Autodesk Inventor part; units mm, degrees
ref_plane "YZ Plane" through (0, 0, 0) normal (1, 0, 0) x (0, 1, 0)
ref_plane "XZ Plane" through (0, 0, 0) normal (0, 1, 0) x (-1, 0, 0)
ref_plane "XY Plane" through (0, 0, 0) normal (0, 0, 1) x (1, 0, 0)
sketch "Эскиз1" plane through (0, 0, 0) normal (1, 0, 0) x (0, 1, 0)
  circle A0 centre (8.3565, 10.4457) radius 25
  point P0 (0, 0)
  dimension "d0" = 50
extrude "Выдавливание1" add sketch "Эскиз1" along normal blind 15
sketch "Эскиз2" plane through (0, 8.3565, 10.4457) normal (-1, 0, 0) x (0, 0, 1)
  circle A0 centre (0, 0) radius 22.5
  point P0 (-10.4457, -8.3565)
  dimension "d3" = 45
extrude "Выдавливание2" cut sketch "Эскиз2" against normal blind 5
sketch "Эскиз3" plane through (15, 8.3565, 10.4457) normal (1, 0, 0) x (0, 0, -1)
  circle A0 centre (0, 0) radius 22.5
  point P0 (10.4457, -8.3565)
  dimension "d6" = 45
extrude "Выдавливание3" cut sketch "Эскиз3" against normal blind 5
sketch "Эскиз7" plane through (5, 8.3565, 10.4457) normal (-1, 0, 0) x (0, 0, 1)
  circle A0 centre (0, 0) radius 5
  line L0 (5, 0) -> (-5, 0)
  line L1 (-5, 0) -> (-5, 30.8448)
  line L2 (-5, 30.8448) -> (5, 30.8448)
  line L3 (5, 30.8448) -> (5, 0)
  line L4 (5, 0) -> (-5, 0)
  line L5 (-5, 0) -> (-5, -27.2335)
  line L6 (-5, -27.2335) -> (5, -27.2335)
  line L7 (5, -27.2335) -> (5, 0)
  line L8 (0, -5) -> (31.8043, -5)
  line L9 (31.8043, -5) -> (31.8043, 5)
  line L10 (31.8043, 5) -> (0, 5)
  line L11 (0, 5) -> (0, -5)
  line L12 (0, -5) -> (-27.8953, -5)
  line L13 (-27.8953, -5) -> (-27.8953, 5)
  line L14 (-27.8953, 5) -> (0, 5)
  line L15 (0, 5) -> (0, -5)
  circle A1 centre (0, 0) radius 22.5
  circle A2 centre (0, 0) radius 17.5
  point P0 (-10.4457, -8.3565)
  point P1 (5, -16.7705)
  point P2 (16.7705, -5)
  point P3 (5, -5)
  point P4 (-16.7705, -5)
  point P5 (-5, -16.7705)
  point P6 (-5, -5)
  point P7 (16.7705, 5)
  point P8 (5, 16.7705)
  point P9 (5, 5)
  point P10 (-5, 16.7705)
  point P11 (-16.7705, 5)
  point P12 (-5, 5)
  dimension "d13" = 10
  dimension "d14" = 35
extrude "Выдавливание4" cut sketch "Эскиз7" against normal blind 10 contours L3 A2 L10 | L8 A2 L7 | L14 A2 L1 | L5 A2 L12
fillet "Сопряжение1" radius 1 2 edges at (15, -16.6435, 10.4457) (0, -16.6435, 10.4457)
properties part number "колесо" material "Пластик САН"
For this review, take the finished solid that the model builds, in its own axes (mm). A direction names the side the tool comes from. Round coordinates to 2 decimals unless told otherwise and drop trailing zeros. Write each loop counter-clockwise with the first axis right and the second up, starting at its lowest first coordinate (ties: lowest second). Pieces come first, ordered by that corner, then holes. Notation, with made-up numbers: (43, 11.5) -> (56, 11.5) arc R22 cw to (56, 45.5) -> close; hole circle Ø10 at (2.5, 4). An arc over 180 degrees is marked (long way). Use one line per item in the form item = value.
1) Tool access review of faces 5 (the flat face through (0, 1, 32)), 6 (the flat face through (10, 9, 11)), 7 (the flat face through (7, 3.356, 21)), 8 (the cylindrical face through (2.465, -11.605, 20.828)): name each direction out of +Z, -Z, +X, -X, +Y, -Y from which nothing blocks a thin tool from reaching the whole face with its end or side.
Found:
face_5 = +Z, -Z, -X, +Y, -Y
face_6 = +X
face_7 = +X, -X
face_8 = -X
2) Mouldability with a two-part tool opening along Z and no side actions: class faces 1 (the flat face through (15, 1, 32)), 2 (the cylindrical face through (12.54, -13.61, 15.32)), 3 (the cylindrical face through (7.465, -4.103, 22.734)), 4 (the cylindrical face through (7.41, -11.48, 25.66)) as +Z half, -Z half, draft (parallel to the pull), parting line (faces both ways), or undercut.
Found:
face_1 = draft
face_2 = undercut
face_3 = undercut
face_4 = parting line
3) Clearance check with flat-ended pins moving along their axes: pin 1 (2 mm diameter, centred on x = 13.5, z = 29, fed in from +Y); pin 2 (2 mm diameter, centred on x = 3, z = 1, fed in from +Y); pin 3 (5 mm diameter, centred on y = -3.5, z = 2, fed in from +X); pin 4 (6 mm diameter, centred on x = 13, y = 22.5, fed in from +Z). State where each tip first meets the part, or that it passes through.
Found:
pin_1 = 26.16
pin_2 = 31.89
pin_3 = through
pin_4 = 32.82
4) Take a section at D-D, the plane x = 13.25. Write out the cut boundary in (y, z), and give its area (3 significant figures).
Found:
outline = circle Ø50 at (8.36, 10.45); hole circle Ø45 at (8.36, 10.45)
area = 373 mm2
5) Take a section at B-B, the plane y = -1.5. Count the separate pieces of the cut face and the enclosed holes in it, and give its area (3 significant figures).
Found:
separate_pieces = 3
enclosed_holes = 0
area = 189 mm2
6) To check wall thickness, follow L1, parallel to Z at x = 9, y = -5; L2, parallel to X at y = 19, z = -5.5; L3, parallel to Y at x = 7.25, z = 25. State the ranges of each line that lie inside material, in increasing order. Write a range as from..to.
Found:
L1 = -10.69..-0.86, 5.45..15.45, 21.75..31.58
L2 = 5..10
L3 = -11.97..-1.36, 3.36..13.36, 18.07..28.68
7) Take a section at A-A, the plane x = 8.5. Write out the cut boundary in (y, z).
Found:
outline = circle Ø50 at (8.36, 10.45); hole (-8.41, 5.45) arc R17.5 ccw to (3.36, -6.32) -> (3.36, 5.45) -> close; hole (-8.41, 15.45) -> (3.36, 15.45) -> (3.36, 27.22) arc R17.5 ccw to start; hole (13.36, -6.32) arc R17.5 ccw to (25.13, 5.45) -> (13.36, 5.45) -> close; hole (13.36, 15.45) -> (25.13, 15.45) arc R17.5 ccw to (13.36, 27.22) -> close
